Source: three-view drawing plus pictorial views. Frame: mm from the lowest corner of the part. A direction names the side the tool comes from. Round coordinates to 2 decimals unless told otherwise and drop trailing zeros. Loops run counter-clockwise (first coordinate to the right, second up) from the corner with the lowest first, then second, coordinate; pieces in that order, holes last. Notation, with made-up numbers: (28, 16.25) -> (54, 16.25) arc R25 cw to (54, 50.25) -> close; hole circle Ø10 at (7.5, 5.5). An arc over 180 degrees is marked (long way). Answer in a Markdown table with one row per item. Add a question column.
Q1. Reachability of the marked faces 1, 2, 3, 4 and 5 from +Z, -Z, +X, -X, +Y, -Y: full face, straight path, thin tool, end or side. Return the list, or none.
Q2. Section B-B, the plane z = 33. Output: boundary loops of the cut face in (x, y), and give its area (4 significant figures).
Q3. Section A-A, the plane y = 25. Output: boundary loops of the cut face in (x, z).
Q4. Pin query (flat end, axial travel): pin 1 (5 mm diameter, centred on x = 88.5, z = 33, fed in from -Y); pin 2 (20 mm diameter, centred on x = 50, y = 48, fed in from +Z); pin 3 (10 mm diameter, centred on x = 64.5, y = 44, fed in from +Z); pin 4 (1 mm diameter, centred on y = 58.5, z = 44.5, fed in from +X). Return the tip coordinate at first contact, or that it passes through.
Q5. Section C-C, the plane x = 47.5. Output: boundary loops of the cut face in (y, z).
Q6. Ray query, L1, parallel to X at y = 66, z = 54.5; L2, parallel to Y at x = 47.5, z = 60.5; L3, parallel to Z at x = 33, y = 44. Return the intervals inside material, ascending. Write a range as from..to.
Q7. Section D-D, the plane y = 42. Output: boundary loops of the cut face in (x, z), and give its area (3 significant figures).
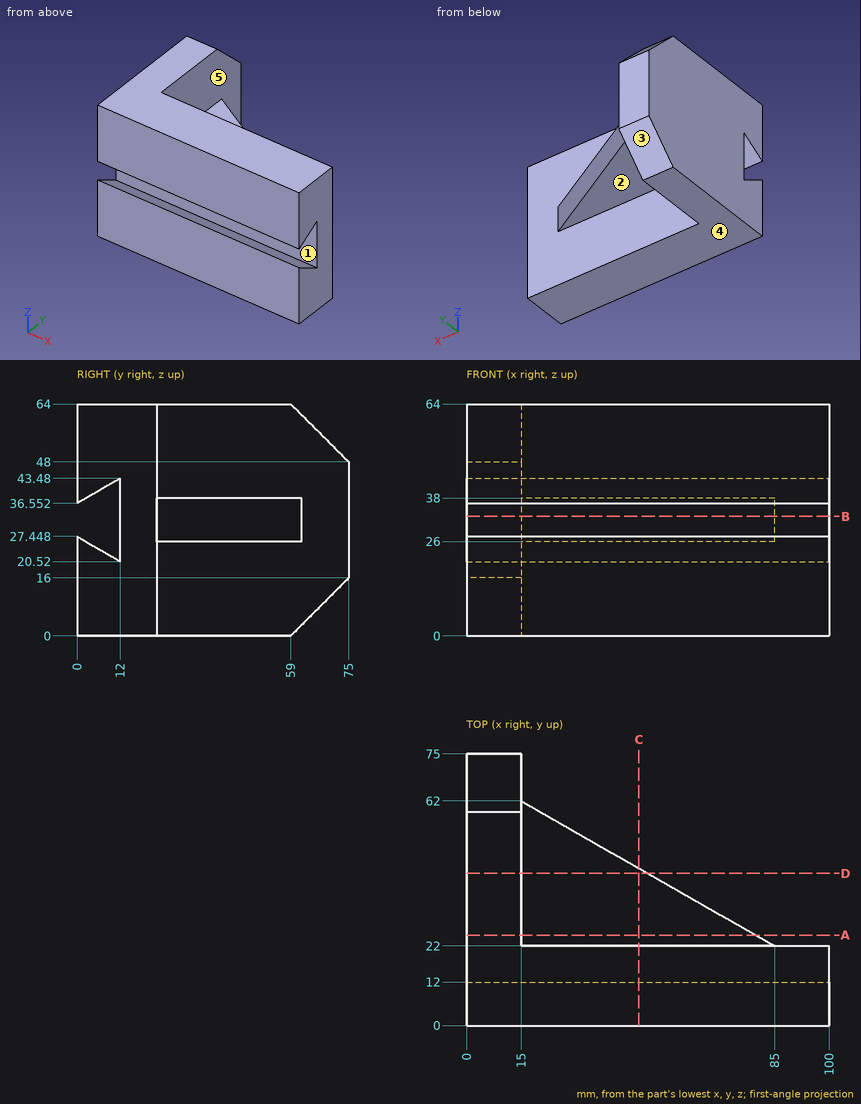
Answer block:
| question | item | result |
|---|---|---|
| 1 | face 1 | +X, -X |
| 1 | face 2 | -Z, +X, +Y |
| 1 | face 3 | -Z, +X, -X, +Y |
| 1 | face 4 | -Z, +X, -X, +Y, -Y |
| 1 | face 5 | +X, +Y |
| 2 | outline | (0, 12) -> (100, 12) -> (100, 22) -> (85, 22) -> (15, 62) -> (15, 75) -> (0, 75) -> close |
| 2 | area | 3,195 mm^2 |
| 3 | outline | (0, 0) -> (15, 0) -> (15, 26) -> (79.75, 26) -> (79.75, 38) -> (15, 38) -> (15, 64) -> (0, 64) -> close |
| 4 | pin 1 | y = 12 |
| 4 | pin 2 | z = 38 |
| 4 | pin 3 | through |
| 4 | pin 4 | x = 15 |
| 5 | outline | (0, 0) -> (22, 0) -> (22, 26) -> (43.43, 26) -> (43.43, 38) -> (22, 38) -> (22, 64) -> (0, 64) -> (0, 36.55) -> (12, 43.48) -> (12, 20.52) -> (0, 27.45) -> close |
| 6 | L1 | 0..15 |
| 6 | L2 | 0..22 |
| 6 | L3 | 26..38 |
| 7 | outline | (0, 0) -> (15, 0) -> (15, 26) -> (50, 26) -> (50, 38) -> (15, 38) -> (15, 64) -> (0, 64) -> close |
| 7 | area | 1,380 mm^2 |
